Part model, mm, in its own coordinate system. Face numbers are marked on the shaded views. A direction names the side the tool comes from. Round coordinates to 2 decimals unless told otherwise and drop trailing zeros. Loops run counter-clockwise (first coordinate to the right, second up) from the corner with the lowest first, then second, coordinate; pieces in that order, holes last.
(1) Tool access for the marked faces 1, 2 and 3: list every direction of +Z, -Z, +X, -X, +Y, -Y with a clear straight run to the whole face (end or side of a thin tool).
(2) Mould opens along Y. For the marked faces 4 and 5 say: +Y half, -Y half, draft (parallel to the pull), parting line (faces both ways), or undercut.
(3) Probe probe 1 along Y at (x, z) = (16, 1.5); probe 2 along Y at (x, z) = (14.5, -1.35); probe 3 along X at (y, z) = (-6, 0.8). List the from-to ranges inside material, lowest first.
(4) Cut at A-A on y = 0. List the corners of the cut face in (x, z), then the cut area to 3 significant figures.
(5) Flat gauge pins, fed straight in: pin 1 (1 mm diameter, centred on y = 7, z = -1.5, fed in from +X); pin 2 (1 mm diameter, centred on y = -16.5, z = 0, fed in from +X); pin 3 (1.7 mm diameter, centred on y = -15, z = 0.5, fed in from -X). Where does each tip first touch, or does it go through?
(6) Cut at B-B on y = 10. Count the separate pieces of the cut face and the enclosed holes in it, then the cut area to 3 significant figures.
from build123d import *

# Parameters (mm, degrees)
F0_R     = 27.94
F1_DEPTH = 1.7907
F4_R     = 2.2225
F5_DEPTH = 1.27


with BuildPart() as f1:
    # F0 (on Top) → F1 (new body, symmetric)
    with BuildSketch(Plane.XY):
        Circle(F0_R)
        with BuildLine():
            ThreePointArc((-19.966928, -6.358759), (-19.597222, -4.089021), (-17.546694, -3.048))
            Line((-17.546694, -3.048), (-14.17857, -3.048))
            ThreePointArc((-14.17857, -3.048), (-12.749232, -3.488335), (-11.815475, -4.656667))
            ThreePointArc((-11.815475, -4.656667), (-8.980256, -8.980256), (-4.656667, -11.815475))
            ThreePointArc((-4.656667, -11.815475), (-3.488335, -12.749232), (-3.048, -14.17857))
            Line((-3.048, -14.17857), (-3.048, -17.546694))
            ThreePointArc((-3.048, -17.546694), (-4.089021, -19.597222), (-6.358759, -19.966928))
            ThreePointArc((-6.358759, -19.966928), (-14.817423, -14.817423), (-19.966928, -6.358759))
        make_face(mode=Mode.SUBTRACT)
        Polygon((6.35, 3.666174), (6.35, -3.666174), (0, -7.332348), (-6.35, -3.666174), (-6.35, 3.666174), (0, 7.332348), align=None, mode=Mode.SUBTRACT)
        with BuildLine():
            Line((3.048, -17.546694), (3.048, -14.17857))
            ThreePointArc((3.048, -14.17857), (3.488335, -12.749232), (4.656667, -11.815475))
            ThreePointArc((4.656667, -11.815475), (8.980256, -8.980256), (11.815475, -4.656667))
            ThreePointArc((11.815475, -4.656667), (12.749232, -3.488335), (14.17857, -3.048))
            Line((14.17857, -3.048), (17.546694, -3.048))
            ThreePointArc((17.546694, -3.048), (19.597222, -4.089021), (19.966928, -6.358759))
            ThreePointArc((19.966928, -6.358759), (14.817423, -14.817423), (6.358759, -19.966928))
            ThreePointArc((6.358759, -19.966928), (4.089021, -19.597222), (3.048, -17.546694))
        make_face(mode=Mode.SUBTRACT)
        with BuildLine():
            ThreePointArc((-3.048, 14.17857), (-3.488335, 12.749232), (-4.656667, 11.815475))
            ThreePointArc((-4.656667, 11.815475), (-8.980256, 8.980256), (-11.815475, 4.656667))
            ThreePointArc((-11.815475, 4.656667), (-12.749232, 3.488335), (-14.17857, 3.048))
            Line((-14.17857, 3.048), (-17.546694, 3.048))
            ThreePointArc((-17.546694, 3.048), (-19.597222, 4.089021), (-19.966928, 6.358759))
            ThreePointArc((-19.966928, 6.358759), (-14.817423, 14.817423), (-6.358759, 19.966928))
            ThreePointArc((-6.358759, 19.966928), (-4.089021, 19.597222), (-3.048, 17.546694))
            Line((-3.048, 17.546694), (-3.048, 14.17857))
        make_face(mode=Mode.SUBTRACT)
        with BuildLine():
            Line((3.048, 14.17857), (3.048, 17.546694))
            ThreePointArc((3.048, 17.546694), (4.089021, 19.597222), (6.358759, 19.966928))
            ThreePointArc((6.358759, 19.966928), (14.817423, 14.817423), (19.966928, 6.358759))
            ThreePointArc((19.966928, 6.358759), (19.597222, 4.089021), (17.546694, 3.048))
            Line((17.546694, 3.048), (14.17857, 3.048))
            ThreePointArc((14.17857, 3.048), (12.749232, 3.488335), (11.815475, 4.656667))
            ThreePointArc((11.815475, 4.656667), (8.980256, 8.980256), (4.656667, 11.815475))
            ThreePointArc((4.656667, 11.815475), (3.488335, 12.749232), (3.048, 14.17857))
        make_face(mode=Mode.SUBTRACT)
    extrude(amount=F1_DEPTH, both=True)

    # F2 (on Right) → F3 (revolve, cut)
    with BuildSketch(Plane.YZ):
        Polygon((27.94, 1.7907), (26.67, 0), (27.94, -1.7907), align=None)
    revolve(axis=Axis((0, 0, 0.396406), (0, 0, -1)), mode=Mode.SUBTRACT)

    # F4 (on face) → F5 (join)
    with BuildSketch(Plane.XY.offset(1.7907)):
        Polygon((6.35, 3.666174), (0, 7.332348), (-6.35, 3.666174), (-6.35, -3.666174), (0, -7.332348), (6.35, -3.666174), align=None)
        Circle(F4_R, mode=Mode.SUBTRACT)
    extrude(amount=-F5_DEPTH)


solid = f1.part
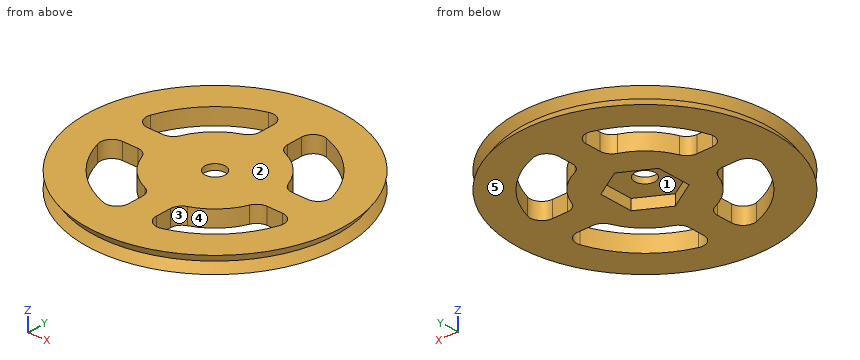
Final values:
1. face 1: -Z
1. face 2: +Z, +X, -X, +Y, -Y
1. face 3: +Z, -Z
2. face 4: undercut
2. face 5: draft
3. probe 1: y = -22.65 to -13.53, -3.05 to 3.05, 13.53 to 22.65
3. probe 2: y = -23.52 to -15.13, -3.05 to 3.05, 15.13 to 23.52
3. probe 3: x = -26.57 to -20.05, -11.19 to 11.19, 20.05 to 26.57
4. outline: (-27.94, -1.79) - (-6.35, -1.79) - (-6.35, 0.52) - (-2.22, 0.52) - (-2.22, 1.79) - (-27.94, 1.79) - (-26.67, 0) - close; (2.22, 0.52) - (6.35, 0.52) - (6.35, -1.79) - (27.94, -1.79) - (26.67, 0) - (27.94, 1.79) - (2.22, 1.79) - close
4. area: 161 mm2
5. pin 1: stops at x = 27.15
5. pin 2: stops at x = 21.54
5. pin 3: stops at x = -23.38
6. separate pieces: 3
6. enclosed holes: 0
6. area: 106 mm2
